```python
from build123d import *

# Parameters (mm, degrees)
SKETCH1_R           = 1.5
SKETCH1_R_2         = 6
SKETCH1_R_3         = 10
BOSS_EXTRUDE1_DEPTH = 4
CUT_EXTRUDE1_DEPTH  = 25


with BuildPart() as part:
    # Sketch1 → Boss-Extrude1 (new body)
    with BuildSketch(Plane(origin=(0, 0, 0), x_dir=(1, 0, 0), z_dir=(0, 1, 0))):
        with BuildLine():
            Line((-50, -39.5), (50, -39.5))
            ThreePointArc((50, -39.5), (57.071067812, -36.571067812), (60, -29.5))
            Line((60, -29.5), (60, 29.5))
            ThreePointArc((60, 29.5), (57.071067812, 36.571067812), (50, 39.5))
            Line((50, 39.5), (-50, 39.5))
            ThreePointArc((-50, 39.5), (-57.071067812, 36.571067812), (-60, 29.5))
            Line((-60, 29.5), (-60, -29.5))
            ThreePointArc((-60, -29.5), (-57.071067812, -36.571067812), (-50, -39.5))
        make_face()
        with Locations(Location((40, 35.5, 0), (0, 0, 270))):
            Circle(SKETCH1_R, mode=Mode.SUBTRACT)
        with Locations(Location((45, 0, 0), (0, 0, 270))):
            Circle(SKETCH1_R_2, mode=Mode.SUBTRACT)
        with Locations(Location((30, 19.45, 0), (0, 0, 270))):
            Circle(SKETCH1_R_3, mode=Mode.SUBTRACT)
        with Locations(Location((30, -19.45, 0), (0, 0, 270))):
            Circle(SKETCH1_R_3, mode=Mode.SUBTRACT)
        with Locations(Location((0, 0, 0), (0, 0, 270))):
            Circle(SKETCH1_R_3, mode=Mode.SUBTRACT)
        with Locations(Location((-30, -19.45, 0), (0, 0, 270))):
            Circle(SKETCH1_R_3, mode=Mode.SUBTRACT)
        with Locations(Location((-46, 35.5, 0), (0, 0, 270))):
            Circle(SKETCH1_R, mode=Mode.SUBTRACT)
        with Locations(Location((-46, -22.5, 0), (0, 0, 270))):
            Circle(SKETCH1_R, mode=Mode.SUBTRACT)
        with Locations(Location((-45, 0, 0), (0, 0, 270))):
            Circle(SKETCH1_R_2, mode=Mode.SUBTRACT)
        with Locations(Location((-30, 19.45, 0), (0, 0, 270))):
            Circle(SKETCH1_R_3, mode=Mode.SUBTRACT)
    extrude(amount=BOSS_EXTRUDE1_DEPTH)

    # Sketch2 → Cut-Extrude1 (cut)
    with BuildSketch(Plane(origin=(0, 4, 0), x_dir=(1, 0, 0), z_dir=(0, 1, 0))):
        with BuildLine():
            ThreePointArc((-50.5, 31), (-53.060660172, 32.060660172), (-52, 29.5))
            Line((-52, 29.5), (-52, 31))
            Line((-52, 31), (-50.5, 31))
        make_face()
        with BuildLine():
            Line((-52, 31), (-52, 29.5))
            ThreePointArc((-52, 29.5), (-50.939339828, 29.939339828), (-50.5, 31))
            Line((-50.5, 31), (-52, 31))
        make_face()
        with BuildLine():
            ThreePointArc((-52, -29.5), (-53.060660172, -32.060660172), (-50.5, -31))
            Line((-50.5, -31), (-52, -31))
            Line((-52, -31), (-52, -29.5))
        make_face()
        with BuildLine():
            Line((-52, -31), (-50.5, -31))
            ThreePointArc((-50.5, -31), (-50.939339828, -29.939339828), (-52, -29.5))
            Line((-52, -29.5), (-52, -31))
        make_face()
        with BuildLine():
            ThreePointArc((52, -29.5), (50.939339828, -29.939339828), (50.5, -31))
            Line((50.5, -31), (52, -31))
            Line((52, -31), (52, -29.5))
        make_face()
        with BuildLine():
            Line((52, -31), (50.5, -31))
            ThreePointArc((50.5, -31), (52, -32.5), (53.5, -31))
            ThreePointArc((53.5, -31), (53.060660172, -29.939339828), (52, -29.5))
            Line((52, -29.5), (52, -31))
        make_face()
        with BuildLine():
            ThreePointArc((50.5, 31), (50.939339828, 29.939339828), (52, 29.5))
            Line((52, 29.5), (52, 31))
            Line((52, 31), (50.5, 31))
        make_face()
        with BuildLine():
            Line((52, 31), (52, 29.5))
            ThreePointArc((52, 29.5), (53.060660172, 29.939339828), (53.5, 31))
            ThreePointArc((53.5, 31), (52, 32.5), (50.5, 31))
            Line((50.5, 31), (52, 31))
        make_face()
    extrude(amount=-CUT_EXTRUDE1_DEPTH, mode=Mode.SUBTRACT)


solid = part.part
```
For this review, take the finished solid that the model builds, in its own axes (mm). Coordinates: 2 decimals unless noted, no trailing zeros. Write each loop counter-clockwise with the first axis right and the second up, starting at its lowest first coordinate (ties: lowest second). Pieces come first, ordered by that corner, then holes. Notation, with made-up numbers: (65.5, 88) - (111.5, 88) arc R16 cw to (111.5, 96) - close; hole circle Ø6 at (83.25, -33). An arc over 180 degrees is marked (long way). Answer in a Markdown table with one row per item. Add a question column.
Q1. We need section B-B, the plane y = 2.65. Count the separate pieces of the cut face and the enclosed holes in it, and give its area (3 significant figures).
Q2. Draft analysis for pull direction X (two halves, no side actions). For faces 1 (the flat face through (-14, 4, -1)), 2 (the cylindrical face through (56.99, 1.97, 36.65)), 3 (the cylindrical face through (-50.857, 1.972, -1.301)), state which applies: +X half, -X half, draft (parallel to the pull), parting line (faces both ways), or undercut.
Q3. For probe 1 along X at (y, z) = (1.1, -19); probe 2 along Z at (x, y) = (8, 2.55); probe 3 along Z at (x, y) = (36.5, 0.2), list the stretches that pass through material, from the lowest coordinate up.
Q4. We need section A-A, the plane z = -19.45. State the section outline as (x, y) points.
Q5. For P1, Ø2.5, axis at x = 40, z = -35.5, coming from the +Y side; P2, Ø3.5, axis at x = -52, z = -31, coming from the -Y side, all flat-tipped, find the tip position at first contact; note any pin that passes through.
Q6. We need section D-D, the plane z = -4.5. State the section outline as (x, y) points, and give its area (3 significant figures).
Q7. We need section C-C, the plane x = -7.5. State the section outline as (y, z) points.
Answer list:
| question | item | result |
|---|---|---|
| 1 | separate pieces | 1 |
| 1 | enclosed holes | 14 |
| 1 | area | 7,550 mm2 |
| 2 | face 1 | draft |
| 2 | face 2 | +X half |
| 2 | face 3 | undercut |
| 3 | probe 1 | x = -60 to -39.99, -20.01 to 20.01, 39.99 to 60 |
| 3 | probe 2 | z = -39.5 to -6, 6 to 39.5 |
| 3 | probe 3 | z = -39.5 to -27.05, -11.85 to 11.85, 27.05 to 39.5 |
| 4 | outline | (-60, 0) - (-40, 0) - (-40, 4) - (-60, 4) - close; (-20, 0) - (20, 0) - (20, 4) - (-20, 4) - close; (40, 0) - (60, 0) - (60, 4) - (40, 4) - close |
| 5 | P1 | passes through |
| 5 | P2 | stops at y = 0 |
| 6 | outline | (-60, 0) - (-48.97, 0) - (-48.97, 4) - (-60, 4) - close; (-41.03, 0) - (-8.93, 0) - (-8.93, 4) - (-41.03, 4) - close; (8.93, 0) - (41.03, 0) - (41.03, 4) - (8.93, 4) - close; (48.97, 0) - (60, 0) - (60, 4) - (48.97, 4) - close |
| 6 | area | 345 mm2 |
| 7 | outline | (0, -39.5) - (4, -39.5) - (4, -6.61) - (0, -6.61) - close; (0, 6.61) - (4, 6.61) - (4, 39.5) - (0, 39.5) - close |
